```python
from build123d import *

# Parameters (mm, degrees)
SKETCH_3_W          = 1.5
SKETCH_3_H          = 12
CUT_EXTRUDE_1_DEPTH = 1


with BuildPart() as part:
    # 草图2 → 旋转1 (revolve)
    with BuildSketch(Plane(origin=(0, 0, 0), x_dir=(0, 0, -1), z_dir=(1, 0, 0))):
        Polygon((0, 0), (0, 6), (3, 6), (3, 4), (21, 4), (21, 3), (29, 3), (29, 0), align=None)
    revolve(axis=Axis((0, 0, 0), (0, 0, -1)))

    # 草图3 → 切除-拉伸1 (cut)
    with BuildSketch(Plane.XY):
        Rectangle(SKETCH_3_W, SKETCH_3_H)
    extrude(amount=-CUT_EXTRUDE_1_DEPTH, mode=Mode.SUBTRACT)


solid = part.part
```
The model under review builds one solid part; all positions refer to its coordinate system, in mm. A direction names the side the tool comes from. Round coordinates to 2 decimals unless told otherwise and drop trailing zeros. Loops run counter-clockwise (first coordinate to the right, second up) from the corner with the lowest first, then second, coordinate; pieces in that order, holes last.
Item 1: Clearance check with flat-ended pins moving along their axes: pin 1 Ø3 at (x, z) = (-2, -19.5) entering from -Y; pin 2 Ø0.5 at (y, z) = (0.5, -0.5) entering from +X; pin 3 Ø1.5 at (y, z) = (-3, -21.5) entering from -X. State where each tip first meets the part, or that it passes through.
Determined:
pin 1: stops at y = -3.97
pin 2: stops at x = 5.99
pin 3: stops at x = -3.17
Item 2: Take a section at A-A (x = 2). Write out the cut boundary in (y, z).
Determined:
outline: (-5.66, -3) - (-3.46, -3) - (-3.46, -21) - (-2.24, -21) - (-2.24, -29) - (2.24, -29) - (2.24, -21) - (3.46, -21) - (3.46, -3) - (5.66, -3) - (5.66, 0) - (-5.66, 0) - close
Item 3: For line 1 (Z direction, x = -3.75, y = 0.5); line 2 (X direction, y = 0, z = -8); line 3 (Z direction, x = 3, y = 3.5), list the stretches that pass through material, from the lowest coordinate up.
Determined:
line 1: z = -21 to 0
line 2: x = -4 to 4
line 3: z = -3 to 0
Item 4: Take a section at B-B (y = 0). Write out the cut boundary in (x, z), then the cut area to 4 significant figures.
Determined:
outline: (-6, -3) - (-4, -3) - (-4, -21) - (-3, -21) - (-3, -29) - (3, -29) - (3, -21) - (4, -21) - (4, -3) - (6, -3) - (6, 0) - (0.75, 0) - (0.75, -1) - (-0.75, -1) - (-0.75, 0) - (-6, 0) - close
area: 226.5 mm2
Item 5: For faces 4 (the face through (0.75, -0.1, -0.5)), 5 (the face through (0, -3, -25)), 6 (the face through (-3, 0, 0)), list the 3-axis set-ups (+Z, -Z, +X, -X, +Y, -Y) from which the entire face can be reached by the end or side of a thin tool; tool diameter is ignored.
Determined:
face 4: +Z, +Y, -Y
face 5: -Z
face 6: +Z, +X, -X, +Y, -Y
Item 6: Mouldability with a two-part tool opening along X and no side actions: class faces 1 (the face through (1.802, 5.723, -1.521)), 2 (the face through (-0.75, -0.1, -0.5)), 3 (the face through (0, 0, -29)) as released by +X, released by -X, zero draft, split by the parting line, or undercut.
Determined:
face 1: split by the parting line
face 2: undercut
face 3: zero draft
Item 7: Take a section at D-D (y = -1.5). Write out the cut boundary in (x, z), then the cut area to 3 significant figures.
Determined:
outline: (-5.81, -3) - (-3.71, -3) - (-3.71, -21) - (-2.6, -21) - (-2.6, -29) - (2.6, -29) - (2.6, -21) - (3.71, -21) - (3.71, -3) - (5.81, -3) - (5.81, 0) - (0.75, 0) - (0.75, -1) - (-0.75, -1) - (-0.75, 0) - (-5.81, 0) - close
area: 208 mm2
Item 8: Take a section at C-C (z = -18). Write out the cut boundary in (x, y), then the cut area to 3 significant figures.
Determined:
outline: circle Ø8 at (0, 0)
area: 50.3 mm2
